from build123d import *

# Parameters (mm, degrees)
F0_R     = 40.782092
F1_DEPTH = 119.040735
F3_R     = 16.942627
F4_DEPTH = 32.315634
F5_SIZE  = 12.7


with BuildPart() as f1:
    # F0 (on Top) → F1 (new body)
    with BuildSketch(Plane.XY):
        Circle(F0_R)
    extrude(amount=F1_DEPTH)

    # F3 (on face) → F4 (cut)
    with BuildSketch(Plane.XY.offset(119.040735)):
        Circle(F3_R)
    extrude(amount=-F4_DEPTH, mode=Mode.SUBTRACT)

    # F5
    f5_edges = [f1.edges().sort_by_distance(p)[0] for p in [
        (-40.782092, 0, 119.040735),
    ]]
    chamfer(f5_edges, length=F5_SIZE)


solid = f1.part
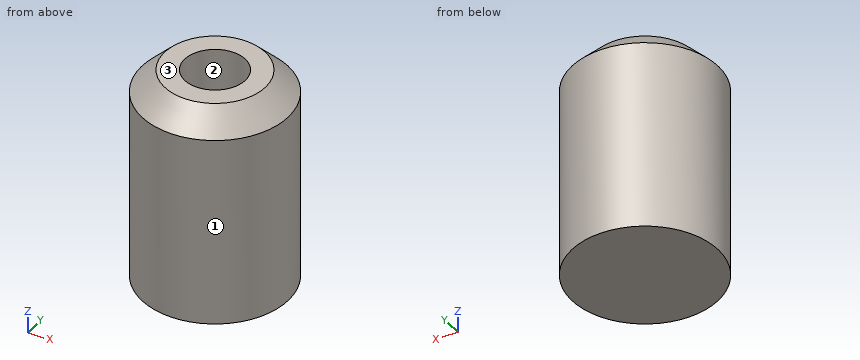
The model under review builds one solid part; all positions refer to its coordinate system, in mm. Face numbers are marked on the shaded views. Round coordinates to 2 decimals unless told otherwise and drop trailing zeros. Loops run counter-clockwise (first coordinate to the right, second up) from the corner with the lowest first, then second, coordinate; pieces in that order, holes last. Notation, with made-up numbers: (-2.75, 0) -> (26.25, 0) arc R23 ccw to (26.25, 39) -> close; hole circle Ø3 at (55, -30.5). An arc over 180 degrees is marked (long way). Write item = value, one per line. Start each with the question number.
Item 1: Take a section at C-C on z = 97. Give the boundary of the cut face in (x, y), plus the area to 3 significant figures.
Item 2: To check wall thickness, follow L1, parallel to Y at x = 0, z = 94; L2, parallel to Z at x = -8, y = -11.5; L3, parallel to X at y = -1, z = 35. State the ranges of each line that lie inside material, in increasing order.
Item 3: Take a section at A-A on x = 0. Give the boundary of the cut face in (y, z), plus the area to 3 significant figures.
Item 4: Take a section at D-D on z = 46. Give the boundary of the cut face in (x, y).
Item 5: Insertion check: pin 1 (12 mm diameter, centred on y = 30.5, z = 88, fed in from -X); pin 2 (1.5 mm diameter, centred on y = -20, z = 17, fed in from -X); pin 3 (2 mm diameter, centred on x = -20.5, z = 53.5, fed in from -Y). Each pin has a flat end and moves straight along its axis. Give the tip position at first contact, or say it passes through.
Item 6: Mouldability with a two-part tool opening along X and no side actions: class the marked faces 1, 2 and 3 as released by +X, released by -X, zero draft, split by the parting line, or undercut.
Result:
q1.outline = circle Ø81.56 at (0, 0); hole circle Ø33.89 at (0, 0)
q1.area = 4,320 mm²
q2.L1 = -40.78 to -16.94, 16.94 to 40.78
q2.L2 = 0 to 86.73
q2.L3 = -40.77 to 40.77
q3.outline = (-40.78, 0) -> (40.78, 0) -> (40.78, 106.34) -> (28.08, 119.04) -> (16.94, 119.04) -> (16.94, 86.73) -> (-16.94, 86.73) -> (-16.94, 119.04) -> (-28.08, 119.04) -> (-40.78, 106.34) -> close
q3.area = 8,450 mm²
q4.outline = circle Ø81.56 at (0, 0)
q5.pin_1 = -32.6
q5.pin_2 = -35.95
q5.pin_3 = -35.82
q6.face_1 = split by the parting line
q6.face_2 = undercut
q6.face_3 = zero draft
